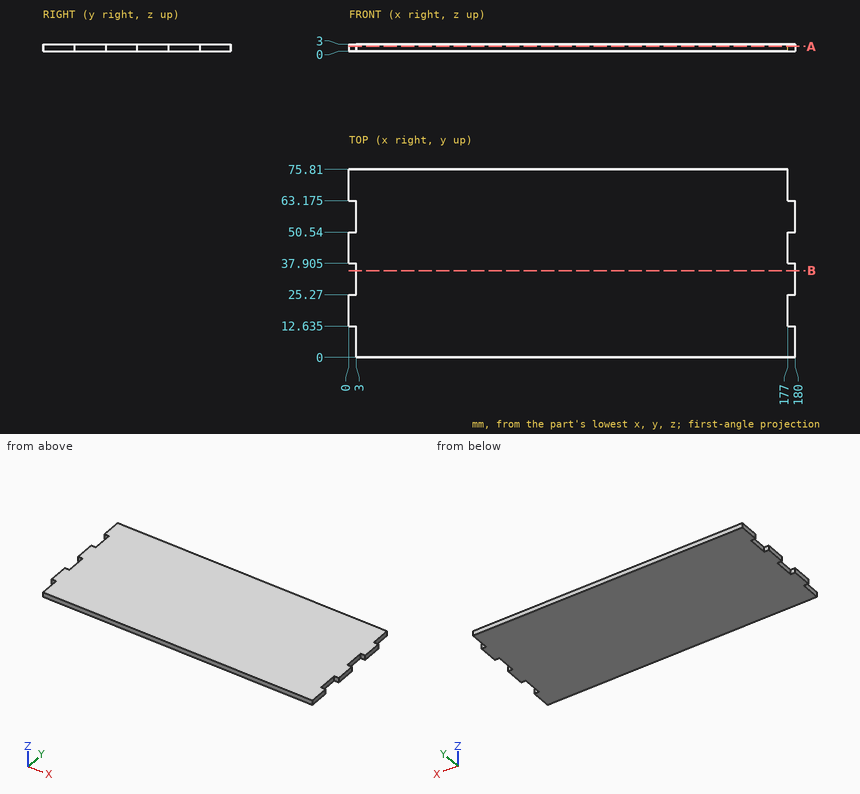
Verification items for this drawing (mm, ordinates from the low corner). Round coordinates to 2 decimals unless told otherwise and drop trailing zeros. Order: outer loops, then holes, each group sorted by start corner. A loop starts at its lowest first (then second) coordinate and runs counter-clockwise, first axis right, second up.
1) Depth check by flat-ended pin: pin 1 (0.9 mm diameter, centred on x = 1, z = 1, fed in from -Y) (3 decimals); pin 2 (0.9 mm diameter, centred on x = 179, z = 1.5, fed in from +Y) (3 decimals). Enter the tip coordinate at first touch or a pass-through.
Geometry says:
pin 1: stops at y = 12.635
pin 2: stops at y = 63.175
2) Cross-section at A-A, the plane z = 2.05. Record the cut outline in (x, y) (3 decimals).
Geometry says:
outline: (0, 12.635) - (3, 12.635) - (3, 0) - (180, 0) - (180, 12.635) - (177, 12.635) - (177, 25.27) - (180, 25.27) - (180, 37.905) - (177, 37.905) - (177, 50.54) - (180, 50.54) - (180, 63.175) - (177, 63.175) - (177, 75.81) - (0, 75.81) - (0, 63.175) - (3, 63.175) - (3, 50.54) - (0, 50.54) - (0, 37.905) - (3, 37.905) - (3, 25.27) - (0, 25.27) - close
3) Material ranges on line 1 (X direction, y = 30, z = 1.1); line 2 (X direction, y = 46.5, z = 1.4), recorded low to high.
Geometry says:
line 1: x = 3 to 180
line 2: x = 0 to 177
4) Cross-section at B-B, the plane y = 35. Record the cut outline in (x, z).
Geometry says:
outline: (3, 0) - (180, 0) - (180, 3) - (3, 3) - close
